The model under review builds one solid part; all positions refer to its coordinate system, in mm. Face numbers are marked on the shaded views. A direction names the side the tool comes from. Coordinates: 2 decimals unless noted, no trailing zeros. Write each loop counter-clockwise with the first axis right and the second up, starting at its lowest first coordinate (ties: lowest second). Pieces come first, ordered by that corner, then holes. Notation, with made-up numbers: (-9, -23) - (39, -23) arc R35 ccw to (39, 10) - close; hole circle Ø6 at (78.5, 67). An arc over 180 degrees is marked (long way). Put each result on its own line as item: value.
from build123d import *
from build123d.topology import SkipClean

# Parameters (mm, degrees)
SKETCH1_R               = 1.2
BOSS_EXTRUDE1_DEPTH     = 1
BOSS_EXTRUDE2_START     = 7.2
BOSS_EXTRUDE2_DEPTH     = 8.2
CHAMFER1_SIZE           = 1
CUT_EXTRUDE1_DEPTH      = 65.659415401
CUT_EXTRUDE1_DEPTH_BACK = 65.659415401
CUT_EXTRUDE2_REACH      = 66.659
SKETCH11_W              = 4.2
SKETCH11_H              = 2
FILLET1_R               = 2
CHAMFER2_SIZE           = 1.7
BOSS_EXTRUDE3_START     = 1
BOSS_EXTRUDE3_DEPTH     = 7


with BuildPart() as part:
    # Sketch1 → Boss-Extrude1 (new body)
    with BuildSketch(Plane(origin=(0, 0, 0), x_dir=(1, 0, 0), z_dir=(0, 1, 0))):
        with BuildLine():
            Line((-60, 0), (-54.5, 0))
            Line((-54.5, 0), (54.5, 0))
            Line((54.5, 0), (60, 0))
            Line((60, 0), (60, 14))
            ThreePointArc((60, 14), (57.363961031, 20.363961031), (51, 23))
            Line((51, 23), (-51, 23))
            ThreePointArc((-51, 23), (-57.363961031, 20.363961031), (-60, 14))
            Line((-60, 14), (-60, 0))
        make_face()
        with Locations(Location((55, 11.43, 0), (0, 0, 270))):
            Circle(SKETCH1_R, mode=Mode.SUBTRACT)
        with Locations(Location((-55, 11.43, 0), (0, 0, 270))):
            Circle(SKETCH1_R, mode=Mode.SUBTRACT)
        with BuildLine():
            Line((-49.887750006, 20.5), (49.887750006, 20.5))
            ThreePointArc((49.887750006, 20.5), (53.580084408, 18.038397435), (52.727888892, 13.683333333))
            ThreePointArc((52.727888892, 13.683333333), (51.958770192, 10.434549723), (54.5, 8.269303874))
            Line((54.5, 8.269303874), (54.5, 2.5))
            Line((54.5, 2.5), (47, 2.5))
            Line((47, 2.5), (47, 0.8))
            Line((47, 0.8), (-47, 0.8))
            Line((-47, 0.8), (-47, 2.5))
            Line((-47, 2.5), (-54.5, 2.5))
            Line((-54.5, 2.5), (-54.5, 8.269303874))
            ThreePointArc((-54.5, 8.269303874), (-51.958770192, 10.434549723), (-52.727888892, 13.683333333))
            ThreePointArc((-52.727888892, 13.683333333), (-53.580084408, 18.038397435), (-49.887750006, 20.5))
        make_face(mode=Mode.SUBTRACT)
    extrude(amount=BOSS_EXTRUDE1_DEPTH)

    # Sketch8 → Boss-Extrude2 (add)
    with SkipClean():  # the faces are left unmerged after this step: merging them gives an invalid solid
        with BuildSketch(Plane(origin=(0, 0, 0), x_dir=(-1, 0, 0), z_dir=(0, -1, 0)).offset(BOSS_EXTRUDE2_START)):
            with BuildLine():
                Line((60, 0), (60, 14))
                ThreePointArc((60, 14), (57.363961031, 20.363961031), (51, 23))
                Line((51, 23), (-51, 23))
                ThreePointArc((-51, 23), (-57.363961031, 20.363961031), (-60, 14))
                Line((-60, 14), (-60, 0))
                Line((-60, 0), (60, 0))
            make_face()
            with BuildLine():
                Line((-59.2, 0.8), (59.2, 0.8))
                Line((59.2, 0.8), (59.2, 14))
                ThreePointArc((59.2, 14), (56.798275606, 19.798275606), (51, 22.2))
                Line((51, 22.2), (-51, 22.2))
                ThreePointArc((-51, 22.2), (-56.798275606, 19.798275606), (-59.2, 14))
                Line((-59.2, 14), (-59.2, 0.8))
            make_face(mode=Mode.SUBTRACT)
        extrude(amount=-BOSS_EXTRUDE2_DEPTH)
    add(part.part.scale(1), mode=Mode.REPLACE)  # the faces are merged on a copy

    # Chamfer1
    chamfer1_edges = [part.edges().sort_by_distance(p)[0] for p in [
        (-56.798275606, 0, -19.798275606),
        (-59.2, 0, -7.4),
        (0, 0, -22.2),
        (56.798275606, 0, -19.798275606),
        (59.2, 0, -7.4),
        (-53.1, 0, -0.8),
        (53.1, 0, -0.8),
    ]]
    chamfer(chamfer1_edges, length=CHAMFER1_SIZE)

    # Sketch9 → Cut-Extrude1 (cut, two sides: drawn at the far end of the back side and taken through both)
    with BuildSketch(Plane(origin=(0, 0, 0), x_dir=(0, 0, -1), z_dir=(1, 0, 0)).offset(-CUT_EXTRUDE1_DEPTH_BACK)):
        Polygon((-2, -7.2), (23, -7.2), (-2, -6.763623377), align=None)
    extrude(amount=CUT_EXTRUDE1_DEPTH + CUT_EXTRUDE1_DEPTH_BACK, mode=Mode.SUBTRACT)

    # Sketch11 → Cut-Extrude2 (cut, up to next)
    with BuildSketch(Plane.XY, mode=Mode.PRIVATE) as cut_extrude2_sk1:
        with Locations((5.35, 0)):
            Rectangle(SKETCH11_W, SKETCH11_H)
    cut_extrude2_tool1 = extrude(cut_extrude2_sk1.sketch, amount=-CUT_EXTRUDE2_REACH, mode=Mode.PRIVATE) & part.part
    add(cut_extrude2_tool1.solids().sort_by_distance((5.35, 0, 0))[0], mode=Mode.SUBTRACT)

    # Fillet1
    fillet1_edges = [part.edges().sort_by_distance(p)[0] for p in [
        (-54.5, 0.5, -8.269303874),
        (-54.5, 0.5, -2.5),
        (54.5, 0.5, -2.5),
        (54.5, 0.5, -8.269303874),
    ]]
    fillet(fillet1_edges, radius=FILLET1_R)

    # Chamfer2
    # the kernel refuses this chamfer: 1.7 mm, written as the material it adds along each edge
    with BuildSketch(Plane(origin=(-47, -5.37186108, -0.8), x_dir=(0.9996219169112968, 0, 0.02749587661058625), z_dir=(0, 1, 0))) as chamfer2_piece_1_section:
        Polygon((CHAMFER2_SIZE * 0.999621916911, CHAMFER2_SIZE * 0.0274958766106), (-CHAMFER2_SIZE * 0.0274958766106, CHAMFER2_SIZE * 0.999621916911), (0, 0), align=None)
    chamfer2_piece_1 = extrude(amount=6.37186108, mode=Mode.PRIVATE)
    chamfer2_piece_1 = split(chamfer2_piece_1, bisect_by=Plane(origin=(-46.825, 0, -2.15), z_dir=(0, 1, 0)), keep=Keep.TOP, mode=Mode.PRIVATE)
    add(chamfer2_piece_1)
    with BuildSketch(Plane(origin=(-47, -5.37186108, -0.8), x_dir=(0.9996219169112968, 0, 0.02749587661058625), z_dir=(0, 1, 0))) as chamfer2_piece_2_section:
        Polygon((CHAMFER2_SIZE * 0.999621916911, CHAMFER2_SIZE * 0.0274958766106), (-CHAMFER2_SIZE * 0.0274958766106, CHAMFER2_SIZE * 0.999621916911), (0, 0), align=None)
    chamfer2_piece_2 = extrude(amount=10.743722159, mode=Mode.PRIVATE)
    chamfer2_piece_2 = split(chamfer2_piece_2, bisect_by=Plane(origin=(-46.296341463, 0, -1.092682927), z_dir=(0, -1, 0)), keep=Keep.TOP, mode=Mode.PRIVATE)
    chamfer2_piece_2 = split(chamfer2_piece_2, bisect_by=Plane(origin=(-46.296341463, -0.530487805, -1.269512195), z_dir=(0, 0.7071067811865476, 0.7071067811865476)), keep=Keep.TOP, mode=Mode.PRIVATE)
    add(chamfer2_piece_2)
    with BuildSketch(Plane(origin=(47, 1, -0.8), x_dir=(0.02749587661058786, 0, -0.9996219169112968), z_dir=(0, -1, 0))) as chamfer2_piece_3_section:
        Polygon((CHAMFER2_SIZE * 0.999621916911, -CHAMFER2_SIZE * 0.0274958766106), (-CHAMFER2_SIZE * 0.0274958766106, -CHAMFER2_SIZE * 0.999621916911), (0, 0), align=None)
    chamfer2_piece_3 = extrude(amount=6.37186108, mode=Mode.PRIVATE)
    chamfer2_piece_3 = split(chamfer2_piece_3, bisect_by=Plane(origin=(46.417200072, 0.023893659, -1.823893659), z_dir=(0, 0.7071067811865476, 0.7071067811865476)), keep=Keep.TOP, mode=Mode.PRIVATE)
    add(chamfer2_piece_3)
    with BuildSketch(Plane(origin=(47, 5.37186108, -0.8), x_dir=(0.02749587661058786, 0, -0.9996219169112968), z_dir=(0, -1, 0))) as chamfer2_piece_4_section:
        Polygon((CHAMFER2_SIZE * 0.999621916911, -CHAMFER2_SIZE * 0.0274958766106), (-CHAMFER2_SIZE * 0.0274958766106, -CHAMFER2_SIZE * 0.999621916911), (0, 0), align=None)
    chamfer2_piece_4 = extrude(amount=10.743722159, mode=Mode.PRIVATE)
    chamfer2_piece_4 = split(chamfer2_piece_4, bisect_by=Plane(origin=(46.825, 0, -2.15), z_dir=(0, 1, 0)), keep=Keep.TOP, mode=Mode.PRIVATE)
    chamfer2_piece_4 = split(chamfer2_piece_4, bisect_by=Plane(origin=(46.825, 0.2625, -2.0625), z_dir=(0, -0.7071067811865476, -0.7071067811865476)), keep=Keep.TOP, mode=Mode.PRIVATE)
    add(chamfer2_piece_4)

    # Sketch12 → Boss-Extrude3 (add)
    with BuildSketch(Plane(origin=(0, 0, 0), x_dir=(1, 0, 0), z_dir=(0, 1, 0)).offset(BOSS_EXTRUDE3_START)):
        with BuildLine():
            Line((-60, 0), (-61.8, 1.8))
            Line((-61.8, 1.8), (-61.8, 14))
            ThreePointArc((-61.8, 14), (-58.636753237, 21.636753237), (-51, 24.8))
            Line((-51, 24.8), (-35.1906155, 24.8))
            ThreePointArc((-35.1906155, 24.8), (-33.11319707, 25.556118473), (-32.007825811, 27.470677654))
            Line((-32.007825811, 27.470677654), (-26.575692405, 58.277837084))
            Line((-26.575692405, 58.277837084), (-25, 58))
            Line((-25, 58), (-30.266576735, 28.131759112))
            ThreePointArc((-30.266576735, 28.131759112), (-31.976677452, 25.169777784), (-35.1906155, 24))
            Line((-35.1906155, 24), (-51, 24))
            ThreePointArc((-51, 24), (-58.071067812, 21.071067812), (-61, 14))
            Line((-61, 14), (-61, 3.5))
            ThreePointArc((-61, 3.5), (-60.5, 3), (-60, 3.5))
            Line((-60, 3.5), (-60, 0))
        make_face()
    boss_extrude3 = extrude(amount=-BOSS_EXTRUDE3_DEPTH)

    # Mirror2: Boss-Extrude3 across plane
    add(boss_extrude3.mirror(Plane(origin=(0, 0, 0), x_dir=(0, 0, 1), z_dir=(1, 0, 0))))


solid = part.part
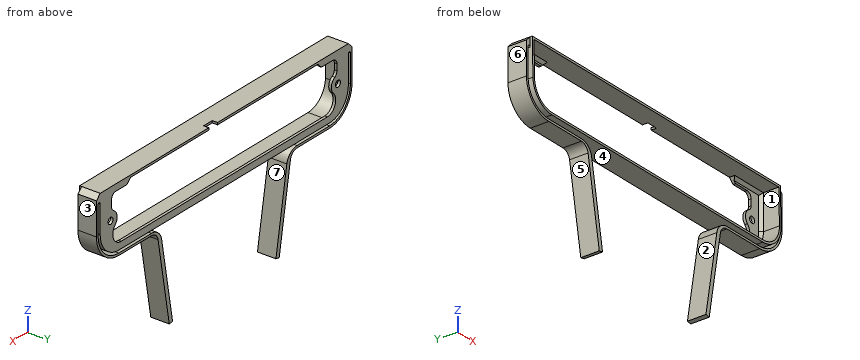
1. Consider section B-B on x = -40. State the section outline as (y, z) points, plus the area to 3 significant figures.
Determined:
outline: (-7.2, -23) - (1, -23) - (1, -20.5) - (0, -20.5) - (0, -21.2) - (-1, -22.2) - (-7.19, -22.2) - close; (-6.81, -0.8) - (1, -0.8) - (1, 0) - (-6.8, 0) - close; (-6, -24.8) - (1, -24.8) - (1, -24) - (-6, -24) - close
area: 20.6 mm^2
2. To check wall thickness, follow probe 1 along Z at (x, y) = (-35, -5); probe 2 along X at (y, z) = (-3.75, -9); probe 3 along X at (y, z) = (0.3, -11.43). State the ranges of each line that lie inside material, in increasing order.
Determined:
probe 1: z = -24.81 to -24, -23 to -22.2, -0.8 to 0
probe 2: x = -61.8 to -61, -60 to -59.2, 59.2 to 60, 61 to 61.8
probe 3: x = -61.8 to -61, -60 to -56.2, -53.8 to -51.8, 51.8 to 53.8, 56.2 to 60, 61 to 61.8
3. For pin 1 Ø0.8 at (x, y) = (48.5, 0.5) entering from -Z; pin 2 Ø18.5 at (x, z) = (-47, -42) entering from -Y; pin 3 Ø2 at (y, z) = (-1, -36.5) entering from -X; pin 4 Ø3 at (x, z) = (-55, -11.43) entering from -Y, all flat-tipped, find the tip position at first contact; note any pin that passes through.
Determined:
pin 1: stops at z = -24.8
pin 2: passes through
pin 3: stops at x = -30.59
pin 4: stops at y = 0
4. Consider section A-A on x = -9. State the section outline as (y, z) points, plus the area to 3 significant figures.
Determined:
outline: (-7.2, -23) - (1, -23) - (1, -20.5) - (0, -20.5) - (0, -21.2) - (-1, -22.2) - (-7.19, -22.2) - close; (-6.81, -0.8) - (1, -0.8) - (1, 0) - (-6.8, 0) - close
area: 15.0 mm^2
5. The part is to be moulded in two halves that separate along Z. For the marked faces 4, 5, 6 and 7, say which applies: +Z half, -Z half, draft (parallel to the pull), parting line (faces both ways), or undercut.
Determined:
face 4: undercut
face 5: -Z half
face 6: draft
face 7: undercut
6. Machinability: for the marked faces 1, 2 and 3, which of the approach directions +Z, -Z, +X, -X, +Y, -Y give a long, thin tool a straight path to every point of the face, cutting with its end or side? Answer none if there is none.
Determined:
face 1: -Y
face 2: +Y, -Y
face 3: +Z, -Z, +X, +Y, -Y
